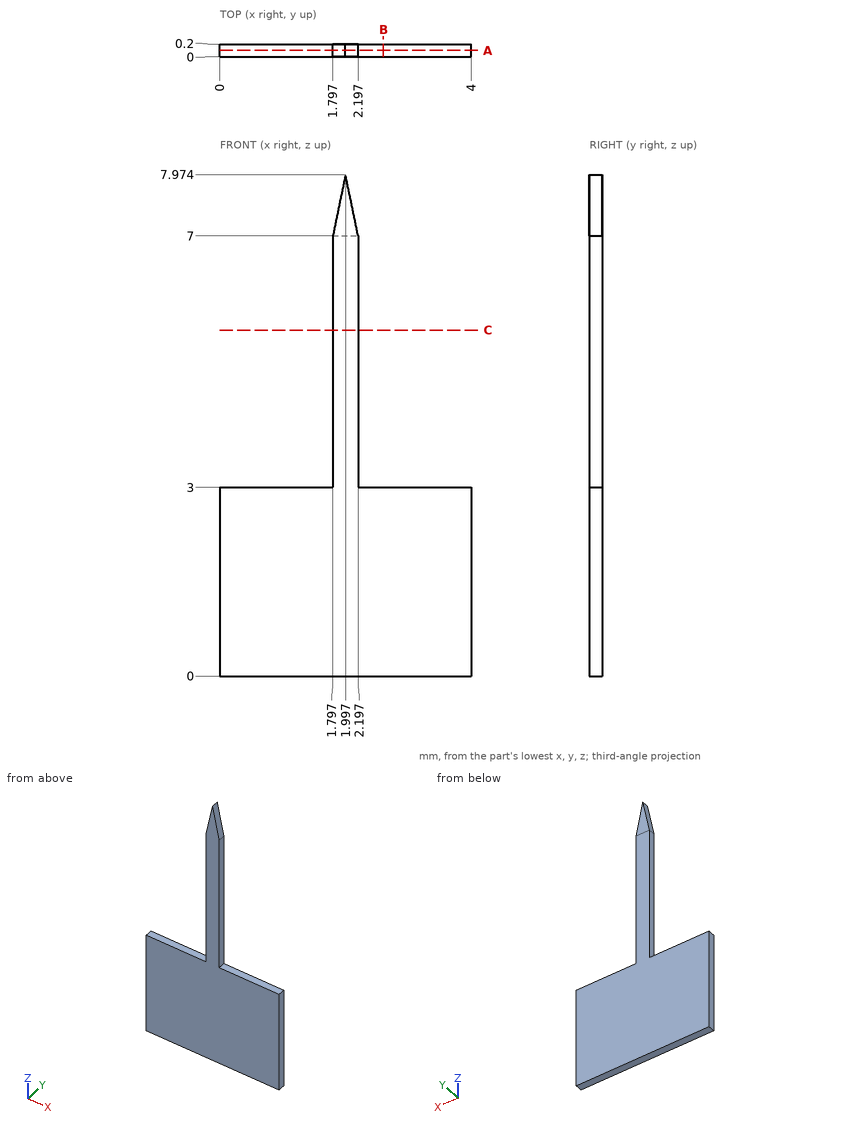
Print and shaded views of the part. All mm, measured from the part's lowest x, y and z. Give positions to 0.01 mm unless a question says otherwise; leave off trailing zeros. Write each loop counter-clockwise with the first axis right and the second up, starting at its lowest first coordinate (ties: lowest second). Pieces come first, ordered by that corner, then holes. Notation, with made-up numbers: (73, 89) - (86, 89) arc R22 cw to (86, 97) - close; hole circle Ø11 at (64.5, 25). An arc over 180 degrees is marked (long way). One line per question, with ' | ' between items. Start each with the question number.
(1) Slice it at C-C on z = 5.5. Write the cut outline in (x, y).
(2) Slice it at A-A on y = 0.1. Write the cut outline in (x, z), plus the area to 3 significant figures.
(3) Slice it at B-B on x = 2.6. Write the cut outline in (y, z).
(4) Wall check: line 1 along Z through (x, y) = (0.45, 0.1); line 2 along X through (y, z) = (0.15, 3.25). Give the ranges that are in metal, low to high. Write a range as from..to.
Results below:
1) outline: (1.8, 0) - (2.2, 0) - (2.2, 0.2) - (1.8, 0.2) - close
2) outline: (0, 0) - (4, 0) - (4, 3) - (2.2, 3) - (2.2, 7) - (2, 7.97) - (1.8, 7) - (1.8, 3) - (0, 3) - close | area: 13.8 mm^2
3) outline: (0, 0) - (0.2, 0) - (0.2, 3) - (0, 3) - close
4) line 1: 0..3 | line 2: 1.8..2.2
